The model under review builds one solid part; all positions refer to its coordinate system, in mm. Face numbers are marked on the shaded views. A direction names the side the tool comes from. Give positions to 0.01 mm unless a question says otherwise; leave off trailing zeros. Write each loop counter-clockwise with the first axis right and the second up, starting at its lowest first coordinate (ties: lowest second). Pieces come first, ordered by that corner, then holes.
Autodesk Inventor part; units mm, degrees
ref_plane "YZ Plane" through (0, 0, 0) normal (1, 0, 0) x (0, 1, 0)
ref_plane "XZ Plane" through (0, 0, 0) normal (0, 1, 0) x (-1, 0, 0)
ref_plane "XY Plane" through (0, 0, 0) normal (0, 0, 1) x (1, 0, 0)
sketch "Sketch1" plane through (0, 0, 0) normal (0, 0, 1) x (1, 0, 0)
  circle A0 centre (0, 0) radius 57.5
  line L0 (0, 0) -> (0, 22.225)
  circle A1 centre (0, 0) radius 60.5
  line L1 (60.5, 0) -> (60.5, 20)
  line L2 (60.5, 0) -> (80.5, 0) construction
  line L3 (-60.5, 0) -> (-60.5, 20)
  line L4 (-60.5, 0) -> (-40.5, 0) construction
  line L5 (-76.5, 37.5) -> (-44.5, 37.5)
  line L6 (-44.5, 37.5) -> (-44.5, 2.5)
  line L7 (-44.5, 2.5) -> (-76.5, 2.5)
  line L8 (-76.5, 2.5) -> (-76.5, 37.5)
  line L9 (-76.5, 37.5) -> (-44.5, 2.5) construction
  line L10 (-44.5, 37.5) -> (-76.5, 2.5) construction
  line L11 (44.5, 37.5) -> (76.5, 37.5)
  line L12 (76.5, 37.5) -> (76.5, 2.5)
  line L13 (76.5, 2.5) -> (44.5, 2.5)
  line L14 (44.5, 2.5) -> (44.5, 37.5)
  line L15 (44.5, 37.5) -> (76.5, 2.5) construction
  line L16 (76.5, 37.5) -> (44.5, 2.5) construction
  point P0 (-57.4456, 2.5)
  point P1 (57.4456, 2.5)
  point P2 (47.4763, 37.5)
  point P3 (-47.4763, 37.5)
  dimension "d0" = 115
  dimension "d27" = 121
  dimension "d28" = 20
  dimension "d29" = 90
  dimension "d30" = 20
  dimension "d31" = 90
  dimension "d32" = 32
  dimension "d33" = 35
  dimension "d34" = 32
  dimension "d35" = 35
extrude "Extrusion1" add sketch "Sketch1" along normal mid plane 20 contours A0 L14 L11 A1 L13 | L7 A1 L5 L6 A0 | A0 L6 L5 A1 L11 L14 | A1 L11 L12 L13 | L7 L8 L5 A1
sketch "Sketch5" plane through (-76.5, 37.5, 10) normal (0, 1, 0) x (1, 0, 0)
  line L0 (0, 0) -> (0, 20)
  line L1 (0, 10) -> (3, 10)
  line L2 (3, 10) -> (8, 10)
  line L3 (13.75, -5) -> (2.25, -5)
  line L4 (2.25, -5) -> (2.25, 25)
  line L5 (2.25, 25) -> (13.75, 25)
  line L6 (13.75, 25) -> (13.75, -5)
  line L7 (13.75, -5) -> (2.25, 25) construction
  line L8 (2.25, -5) -> (13.75, 25) construction
  point P0 (76.5, 10)
  dimension "d36" = 3
  dimension "d37" = 5
  dimension "d38" = 11.5
  dimension "d39" = 30
extrude "Extrusion5" cut sketch "Sketch5" against normal blind 13
sketch "Sketch6" plane through (-76.5, 24.5, 10) normal (0, 1, 0) x (1, 0, 0)
  line L0 (13.75, 0) -> (2.25, 0)
  line L1 (13.75, 20) -> (13.75, 0)
  line L2 (2.25, 20) -> (13.75, 20)
  line L3 (2.25, 0) -> (2.25, 20)
  line L4 (8, 0) -> (8, 8)
  line L5 (13.75, 0) -> (2.25, 0)
  line L6 (2.25, 0) -> (2.25, 16)
  line L7 (2.25, 16) -> (13.75, 16)
  line L8 (13.75, 16) -> (13.75, 0)
  line L9 (13.75, 0) -> (2.25, 16) construction
  line L10 (2.25, 0) -> (13.75, 16) construction
  point P0 (76.5, 10)
  point P1 (13.75, 16)
  point P2 (2.25, 16)
  dimension "d42" = 8
  dimension "d43" = 11.5
  dimension "d44" = 16
extrude "Extrusion6" cut sketch "Sketch6" against normal blind 15 contours L0 L3 L7 L1
sketch "Sketch7" plane through (-76.5, 2.5, 10) normal (-1, 0, 0) x (0, 0, 1)
  line L0 (0, 35) -> (0, 0)
  line L1 (-16, 7) -> (0, 7)
  line L2 (0, 35) -> (-16, 35)
  line L3 (-16, 35) -> (-16, 7)
  line L4 (-16, 7) -> (0, 7)
  line L5 (0, 7) -> (0, 35)
  line L6 (-16, 7) -> (-14, 7)
  line L7 (-14, 7) -> (-14, 9)
  line L8 (0, 35) -> (-3, 35)
  line L9 (0, 35) -> (-20, 35)
  line L10 (0, 35) -> (3, 35) construction
  line L11 (-3, 35) -> (-3, 32)
  circle A0 centre (-3, 32) radius 1.5
  circle A1 centre (-14, 9) radius 1.5
  point P0 (-10, -2.5)
  dimension "d47" = 16
  dimension "d48" = 28
  dimension "d49" = 2
  dimension "d50" = 2
  dimension "d51" = 90
  dimension "d52" = 3
  dimension "d53" = 180
  dimension "d54" = 3
  dimension "d55" = 3
  dimension "d56" = 3
extrude "Extrusion7" cut sketch "Sketch7" against normal blind 20 contours A0 | A1
mirror "Mirror2" about plane through (0, 0, 0) normal (1, 0, 0) of "Extrusion5", "Extrusion6", "Extrusion7"
chamfer "Chamfer1" distance 5 angle 45 2 edges at (-76.5, 2.5, 0) (76.5, 2.5, 0)
fillet "Fillet1" radius 7 2 edges at (-47.4763, 37.5, 0) (47.4763, 37.5, 0)
chamfer "Chamfer2" distance 5 angle 45 2 edges at (-57.4456, 2.5, 0) (57.4456, 2.5, 0)
sketch "Sketch8" plane through (-76.5, 9.5, 10) normal (0, 1, 0) x (1, 0, 0)
  line L0 (13.75, 0) -> (2.25, 0)
  line L1 (8, 0) -> (8, 3)
  line L2 (13.75, 6) -> (2.25, 6)
  line L3 (2.25, 6) -> (2.25, 0)
  line L4 (2.25, 0) -> (13.75, 0)
  line L5 (13.75, 0) -> (13.75, 6)
  line L6 (13.75, 6) -> (2.25, 0) construction
  line L7 (2.25, 6) -> (13.75, 0) construction
  line L8 (13.75, 3) -> (2.25, 3)
  point P0 (76.5, 10)
  point P1 (13.75, 0)
  dimension "d66" = 3
  dimension "d67" = 11.5
  dimension "d68" = 6
extrude "Extrusion8" cut sketch "Sketch8" against normal blind 20 contours L0 L1 L8 L5 | L0 L3 L8 L1
mirror "Mirror3" about plane through (0, 0, 0) normal (1, 0, 0) of "Extrusion8"
sketch "Sketch9" plane through (0, 0, 10) normal (0, 0, 1) x (1, 0, 0)
  line L0 (-60.325, 74.6125) -> (82.55, 74.6125)
  line L1 (82.55, 74.6125) -> (82.55, -23.8125)
  line L2 (82.55, -23.8125) -> (-60.325, -23.8125)
  line L3 (-60.325, -23.8125) -> (-60.325, 74.6125)
  point P0 (0, 0)
extrude "Extrusion9" cut sketch "Sketch9" against normal blind 30
properties part number "IMPRIMIR SOPORTE"
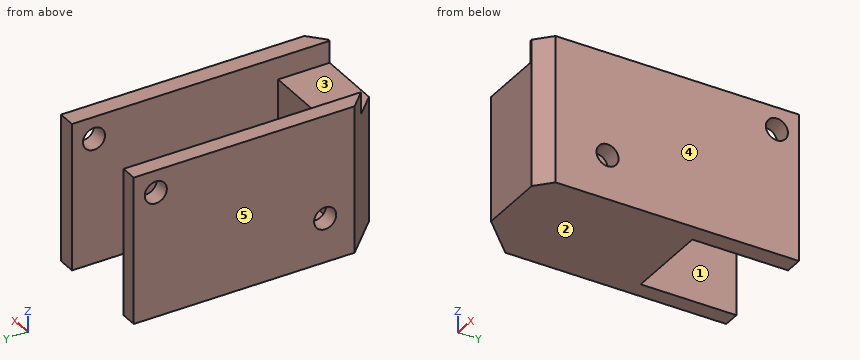
1) The part is to be moulded in two halves that separate along X. For the marked faces 3, 4 and 5, say which applies: +X half, -X half, draft (parallel to the pull), parting line (faces both ways), or undercut.
2) Tool access review of the marked faces 1 and 2: name each direction out of +Z, -Z, +X, -X, +Y, -Y from which nothing blocks a thin tool from reaching the whole face with its end or side.
3) Consider section B-B, the plane y = 34.5. Give the boundary of the cut face in (x, z) (3 decimals), then the cut area to 3 significant figures.
4) Consider section C-C, the plane x = -75.25. Give the boundary of the cut face in (y, z), then the cut area to 3 significant figures.
5) To check wall thickness, follow probe 1 along X at (y, z) = (32, 6) (3 decimals); probe 2 along Y at (x, z) = (-63, 0.25); probe 3 along Z at (x, y) = (-74.95, 11.5). State the ranges of each line that lie inside material, in increasing order.
6) Insertion check: pin 1 (2.5 mm diameter, centred on y = 34.5, z = 7, fed in from -X); pin 2 (2 mm diameter, centred on x = -70.5, z = -8, fed in from +Y); pin 3 (5.5 mm diameter, centred on x = -70, y = 6, fed in from +Z); pin 4 (1 mm diameter, centred on x = -64.5, z = -4, fed in from +Y). Each pin has a flat end and moves straight along its axis. Give the tip position at first contact, or say it passes through.
7) Consider section D-D, the plane y = 25. Give the boundary of the cut face in (x, z) (3 decimals).
8) Consider section A-A, the plane z = -4. Give the boundary of the cut face in (x, y) (3 decimals).
Answer block:
1. face 3: undercut
1. face 4: +X half
1. face 5: -X half
2. face 1: +Z, +Y
2. face 2: -Z, +X, -X, +Y, -Y
3. outline: (-76.5, -10) - (-74.25, -10) - (-74.25, 5.5) - (-76.5, 5.5) - close; (-76.5, 8.5) - (-74.25, 8.5) - (-74.25, 10) - (-76.5, 10) - close; (-62.75, -10) - (-60.325, -10) - (-60.325, 5.5) - (-62.75, 5.5) - close; (-62.75, 8.5) - (-60.325, 8.5) - (-60.325, 10) - (-62.75, 10) - close
3. area: 79.5 mm2
4. outline: (6.25, -10) - (37.5, -10) - (37.5, 10) - (6.25, 10) - close; hole circle Ø3 at (11.5, -4); hole circle Ø3 at (34.5, 7)
4. area: 611 mm2
5. probe 1: x = -76.5 to -74.25, -62.75 to -60.325
5. probe 2: y = 2.5 to 9.5
5. probe 3: z = -10 to -5.5, -2.5 to 10
6. pin 1: passes through
6. pin 2: stops at y = 24.5
6. pin 3: stops at z = 7
6. pin 4: stops at y = 9.5
7. outline: (-76.5, -10) - (-74.25, -10) - (-74.25, 10) - (-76.5, 10) - close; (-62.75, -10) - (-60.325, -10) - (-60.325, 10) - (-62.75, 10) - close
8. outline: (-76.5, 7.5) - (-71.5, 2.5) - (-62.446, 2.5) - (-60.325, 4.444) - (-60.325, 10) - (-62.75, 10) - (-62.75, 9.5) - (-74.25, 9.5) - (-74.25, 10) - (-76.5, 10) - close; (-76.5, 13) - (-74.25, 13) - (-74.25, 37.5) - (-76.5, 37.5) - close; (-62.75, 13) - (-60.325, 13) - (-60.325, 37.5) - (-62.75, 37.5) - close
